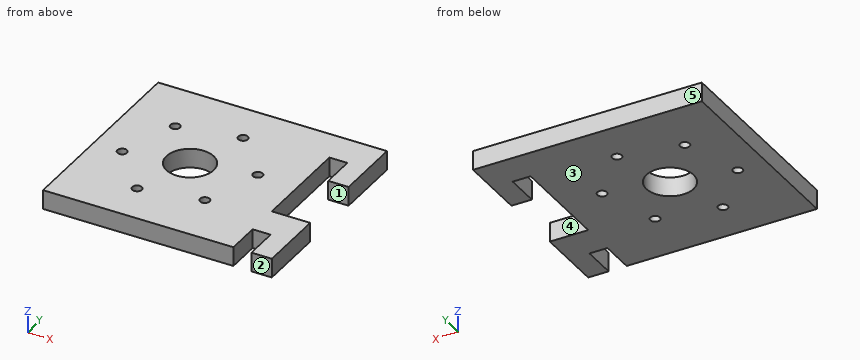
```python
from build123d import *

# Parameters (mm, degrees)
SKETCH1_W           = 57.15
SKETCH1_H           = 50.8
BOSS_EXTRUDE1_DEPTH = 4.800000052
CUT_EXTRUDE4_DEPTH  = 77.614636333
SKETCH7_R           = 5.9
CUT_EXTRUDE6_DEPTH  = 100.346049289
SKETCH10_R          = 1.2
CUT_EXTRUDE9_DEPTH  = 100.346049289
SKETCH11_W          = 4.500000144
SKETCH11_H          = 8.466666667
CUT_EXTRUDE10_DEPTH = 77.614636333
CUT_EXTRUDE11_DEPTH = 77.614636333


with BuildPart() as part:
    # Sketch1 → Boss-Extrude1 (new body)
    with BuildSketch(Plane.XY):
        with Locations((28.575, 25.4)):
            Rectangle(SKETCH1_W, SKETCH1_H)
    extrude(amount=BOSS_EXTRUDE1_DEPTH)

    # Sketch5 → Cut-Extrude4 (cut, through all)
    with BuildSketch(Plane.XY.offset(4.800000052)):
        Polygon((52.349999948, 25.4), (57.15, 16.933333333), (57.15, 33.866666667), align=None)
        Polygon((47.549999896, 16.933333333), (57.15, 16.933333333), (52.349999948, 25.4), align=None)
        Polygon((47.549999896, 33.866666667), (47.549999896, 16.933333333), (52.349999948, 25.4), align=None)
        Polygon((52.349999948, 25.4), (57.15, 33.866666667), (47.549999896, 33.866666667), align=None)
    extrude(amount=-CUT_EXTRUDE4_DEPTH, mode=Mode.SUBTRACT)

    # Sketch7 → Cut-Extrude6 (cut, through all)
    with BuildSketch(Plane(origin=(60.342507963, 78.774229552, 4.800000052), x_dir=(0, 1, 0), z_dir=(0, 0, 1))):
        with Locations(Location((-53.374229552, 38.000051, 0), (0, 0, 270))):
            Circle(SKETCH7_R)
    extrude(amount=-CUT_EXTRUDE6_DEPTH, mode=Mode.SUBTRACT)

    # Sketch10 → Cut-Extrude9 (cut, through all)
    with BuildSketch(Plane(origin=(60.342507963, 78.774229552, 4.800000052), x_dir=(0, 1, 0), z_dir=(0, 0, 1))):
        with Locations(Location((-64.981804426, 27.728040216, 0), (0, 0, 270))):
            Circle(SKETCH10_R)
        with Locations(Location((-56.466264402, 53.188511109, 0), (0, 0, 270))):
            Circle(SKETCH10_R)
        with Locations(Location((-68.073839276, 42.916500326, 0), (0, 0, 270))):
            Circle(SKETCH10_R)
        with Locations(Location((-50.282194703, 22.811590891, 0), (0, 0, 270))):
            Circle(SKETCH10_R)
        with Locations(Location((-38.674619828, 33.083601674, 0), (0, 0, 270))):
            Circle(SKETCH10_R)
        with Locations(Location((-41.766654678, 48.272061784, 0), (0, 0, 270))):
            Circle(SKETCH10_R)
    extrude(amount=-CUT_EXTRUDE9_DEPTH, mode=Mode.SUBTRACT)

    # Sketch11 → Cut-Extrude10 (cut, through all)
    with BuildSketch(Plane.XY.offset(4.800000052)):
        with Locations((49.799999968, 4.233333334)):
            Rectangle(SKETCH11_W, SKETCH11_H)
    extrude(amount=-CUT_EXTRUDE10_DEPTH, mode=Mode.SUBTRACT)

    # Sketch12 → Cut-Extrude11 (cut, through all)
    with BuildSketch(Plane.XY.offset(4.800000052)):
        Polygon((49.799999968, 38.1), (47.549999896, 33.866666667), (52.05000004, 33.866666667), align=None)
        Polygon((47.549999896, 42.333333333), (47.549999896, 33.866666667), (49.799999968, 38.1), align=None)
        Polygon((49.799999968, 38.1), (52.05000004, 33.866666667), (52.05000004, 42.333333333), align=None)
        Polygon((52.05000004, 42.333333333), (47.549999896, 42.333333333), (49.799999968, 38.1), align=None)
    extrude(amount=-CUT_EXTRUDE11_DEPTH, mode=Mode.SUBTRACT)


solid = part.part
```
Build history of the part. All positions in model axes, mm. Face numbers are marked on the shaded views. A direction names the side the tool comes from. Coordinates: 2 decimals unless noted, no trailing zeros. Order: outer loops, then holes, each group sorted by start corner. A loop starts at its lowest first (then second) coordinate and runs counter-clockwise, first axis right, second up.
Item 1: Drill centre lines: L1, parallel to Y at x = 52.5, z = 0.5; L2, parallel to X at y = 37.5, z = 4.1; L3, parallel to Y at x = 18, z = 1.75. Where is each one in solid material? Low to high.
Filled in:
L1: y = 0 to 16.93, 33.87 to 50.8
L2: x = 0 to 10.98, 13.16 to 47.55, 52.05 to 57.15
L3: y = 0 to 9.65, 11.75 to 21.41, 29.39 to 50.8
Item 2: Drop flat-ended pins along their axis: pin 1 Ø1 at (x, y) = (10.5, 33) entering from -Z; pin 2 Ø1.9 at (x, y) = (17.43, 10.7) entering from +Z; pin 3 Ø2.5 at (x, z) = (50, 2) entering from -Y; pin 4 Ø1.5 at (y, z) = (28.5, 2.5) entering from +X. Give the stop position or say it passes through.
Filled in:
pin 1: stops at z = 0
pin 2: passes through
pin 3: stops at y = 8.47
pin 4: stops at x = 47.55
Item 3: Tool access for the marked faces 4 and 5: list every direction of +Z, -Z, +X, -X, +Y, -Y with a clear straight run to the whole face (end or side of a thin tool).
Filled in:
face 4: +Z, -Z, +X
face 5: +Z, -Z, +X, -X, +Y
Item 4: Saw through at B-B on y = 25.4. List the corners of the cut face in (x, z).
Filled in:
outline: (0, 0) - (16.44, 0) - (16.44, 4.8) - (0, 4.8) - close; (28.24, 0) - (47.55, 0) - (47.55, 4.8) - (28.24, 4.8) - close
Item 5: Mould opens along Y. For the marked faces 1, 2 and 3 say: released by +Y, released by -Y, zero draft, split by the parting line, or undercut.
Filled in:
face 1: undercut
face 2: released by -Y
face 3: zero draft
Item 6: Saw through at C-C on z = 1.2. List the corners of the cut face in (x, y).
Filled in:
outline: (0, 0) - (47.55, 0) - (47.55, 8.47) - (52.05, 8.47) - (52.05, 0) - (57.15, 0) - (57.15, 16.93) - (47.55, 16.93) - (47.55, 42.33) - (52.05, 42.33) - (52.05, 33.87) - (57.15, 33.87) - (57.15, 50.8) - (0, 50.8) - close; hole circle Ø2.4 at (7.15, 22.31); hole circle Ø2.4 at (12.07, 37.01); hole circle Ø2.4 at (17.43, 10.7); hole circle Ø11.8 at (22.34, 25.4); hole circle Ø2.4 at (27.26, 40.1); hole circle Ø2.4 at (32.61, 13.79); hole circle Ø2.4 at (37.53, 28.49)
Item 7: Saw through at A-A on x = 53. List the corners of the cut face in (y, z), then the cut area to 3 significant figures.
Filled in:
outline: (0, 0) - (16.93, 0) - (16.93, 4.8) - (0, 4.8) - close; (33.87, 0) - (50.8, 0) - (50.8, 4.8) - (33.87, 4.8) - close
area: 163 mm2
